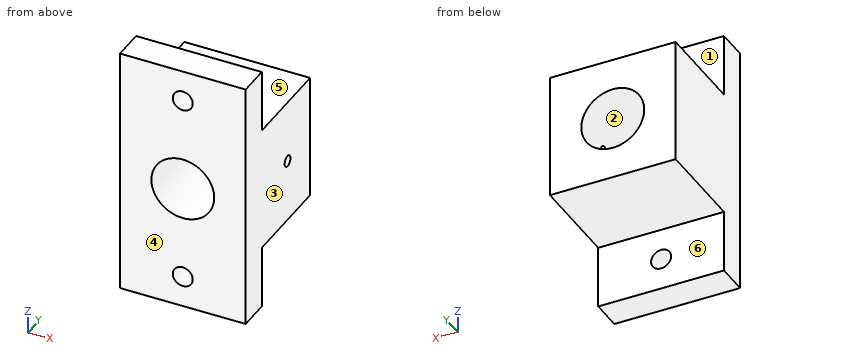
```python
from build123d import *

# Parameters (mm, degrees)
SKETCH1_W                  = 25.4
SKETCH1_H                  = 50.8
BOSS_EXTRUDE1_DEPTH        = 6.35
SKETCH2_W                  = 25.4
SKETCH2_H                  = 25.4
BOSS_EXTRUDE2_DEPTH        = 19.05
SKETCH3_R                  = 6.35
CUT_EXTRUDE1_DEPTH         = 39.1
F_10_32_TAPPED_HOLE1_D     = 4.0386
F_4_40_TAPPED_HOLE1_REACH  = 45.994
F_4_40_TAPPED_HOLE1_BORE_R = 1.1303


with BuildPart() as part:
    # Sketch1 → Boss-Extrude1 (new body)
    with BuildSketch(Plane(origin=(0, 0, 0), x_dir=(1, 0, 0), z_dir=(0, 1, 0))):
        Rectangle(SKETCH1_W, SKETCH1_H)
    extrude(amount=BOSS_EXTRUDE1_DEPTH)

    # Sketch2 → Boss-Extrude2 (add)
    with BuildSketch(Plane(origin=(0, 6.35, 0), x_dir=(1, 0, 0), z_dir=(0, 1, 0))):
        Rectangle(SKETCH2_W, SKETCH2_H)
    extrude(amount=BOSS_EXTRUDE2_DEPTH)

    # Sketch3 → Cut-Extrude1 (cut, through all)
    with BuildSketch(Plane(origin=(0, 25.4, 0), x_dir=(1, 0, 0), z_dir=(0, 1, 0))):
        with Locations(Location((0, 0, 0), (0, 0, 270))):
            Circle(SKETCH3_R)
    extrude(amount=-CUT_EXTRUDE1_DEPTH, mode=Mode.SUBTRACT)

    # #10-32 Tapped Hole1 (through all)
    with Locations(Plane(origin=(0, 6.35, 0), x_dir=(1, 0, 0), z_dir=(0, 1, 0))):
        with Locations((0, 19.05), (0, -19.05)):
            Hole(F_10_32_TAPPED_HOLE1_D / 2)

    # #4-40 Tapped Hole1 bore → #4-40 Tapped Hole1 (cut, up to next)
    with BuildSketch(Plane(origin=(12.7, 0, 0), x_dir=(0, 0, -1), z_dir=(1, 0, 0)), mode=Mode.PRIVATE) as f_4_40_tapped_hole1_sk1:
        with Locations((0, 16.51)):
            Circle(F_4_40_TAPPED_HOLE1_BORE_R)
    f_4_40_tapped_hole1_tool1 = extrude(f_4_40_tapped_hole1_sk1.sketch, amount=-F_4_40_TAPPED_HOLE1_REACH, mode=Mode.PRIVATE) & part.part
    add(f_4_40_tapped_hole1_tool1.solids().sort_by_distance((12.7, 16.51, 0))[0], mode=Mode.SUBTRACT)


solid = part.part
```
Design review of the part built by this model. Coordinates are the model's own, in mm. Face numbers are marked on the shaded views. A direction names the side the tool comes from. Coordinates: 2 decimals unless noted, no trailing zeros. Loops run counter-clockwise (first coordinate to the right, second up) from the corner with the lowest first, then second, coordinate; pieces in that order, holes last. Notation, with made-up numbers: (54.5, 76) - (88.5, 76) arc R14 ccw to (88.5, 85) - close; hole circle Ø10 at (-16.5, -37). An arc over 180 degrees is marked (long way). Use CSV: the item, a comma, the result in double quotes. Start each with the question number.
1) Consider section C-C on z = 0. Write out the cut boundary in (x, y).
2) Consider section B-B on z = 19.05. Write out the cut boundary in (x, y).
3) For pin 1 Ø10 at (x, z) = (1, -18.5) entering from +Y; pin 2 Ø10 at (x, y) = (0, 19.5) entering from -Z; pin 3 Ø11.5 at (x, z) = (0, 0) entering from -Y; pin 4 Ø2 at (x, y) = (3.5, 12) entering from +Z, all flat-tipped, find the tip position at first contact; note any pin that passes through.
4) Consider section D-D on y = 4.5. Write out the cut boundary in (x, z).
5) The part is to be moulded in two halves that separate along X. For the marked faces 1, 2 and 3, say which applies: +X half, -X half, draft (parallel to the pull), parting line (faces both ways), or undercut.
6) Tool access review of the marked faces 4, 5 and 6: name each direction out of +Z, -Z, +X, -X, +Y, -Y from which nothing blocks a thin tool from reaching the whole face with its end or side.
7) Consider section A-A on x = 0. Write out the cut boundary in (y, z), then the cut area to 3 significant figures.
8) Wall thickness on L1, parallel to X at y = 3, z = 19.05; L2, parallel to Y at x = 9, z = 0; L3, parallel to Y at x = 11, z = -13: over which ranges is each line inside the solid? List them lowest first. Write a range as from..to.
Geometry says:
1,outline,"(-12.7, 0) - (-6.35, 0) - (-6.35, 25.4) - (-12.7, 25.4) - close; (6.35, 0) - (12.7, 0) - (12.7, 15.38) - (6.35, 15.38) - close; (6.35, 17.64) - (12.7, 17.64) - (12.7, 25.4) - (6.35, 25.4) - close"
2,outline,"(-12.7, 0) - (-2.02, 0) - (-2.02, 6.35) - (-12.7, 6.35) - close; (2.02, 0) - (12.7, 0) - (12.7, 6.35) - (2.02, 6.35) - close"
3,pin 1,"y = 6.35"
3,pin 2,"z = -12.7"
3,pin 3,"through"
3,pin 4,"z = 12.7"
4,outline,"(-12.7, -25.4) - (12.7, -25.4) - (12.7, 25.4) - (-12.7, 25.4) - close; hole circle Ø12.7 at (0, 0); hole circle Ø4.04 at (0, -19.05); hole circle Ø4.04 at (0, 19.05)"
5,face 1,"draft"
5,face 2,"undercut"
5,face 3,"+X half"
6,face 4,"+Z, -Z, +X, -X, -Y"
6,face 5,"+Z, +X, -X, +Y"
6,face 6,"-Z, +X, -X, +Y"
7,outline,"(0, -25.4) - (6.35, -25.4) - (6.35, -21.07) - (0, -21.07) - close; (0, -17.03) - (6.35, -17.03) - (6.35, -12.7) - (25.4, -12.7) - (25.4, -6.35) - (0, -6.35) - close; (0, 6.35) - (25.4, 6.35) - (25.4, 12.7) - (6.35, 12.7) - (6.35, 17.03) - (0, 17.03) - close; (0, 21.07) - (6.35, 21.07) - (6.35, 25.4) - (0, 25.4) - close"
7,area,"433 mm^2"
8,L1,"-12.7..-2.02, 2.02..12.7"
8,L2,"0..15.38, 17.64..25.4"
8,L3,"0..6.35"
